```python
from build123d import *

# Parameters (mm, degrees)
SKETCH_1_W      = 100
SKETCH_1_H      = 100
SKETCH_1_R      = 1.65
EXTRUDE_1_DEPTH = 4
FILLET_1_R      = 3
SKETCH_2_W      = 9.3
SKETCH_2_H      = 10.3
EXTRUDE_2_DEPTH = 5


with BuildPart() as part:
    # 草图1 → 凸台-拉伸1 (new body)
    with BuildSketch(Plane(origin=(0, 0, 0), x_dir=(1, 0, 0), z_dir=(0, 1, 0))):
        Rectangle(SKETCH_1_W, SKETCH_1_H)
        with Locations(Location((-46, 46, 0), (0, 0, 270))):
            Circle(SKETCH_1_R, mode=Mode.SUBTRACT)
        with Locations(Location((46, 46, 0), (0, 0, 270))):
            Circle(SKETCH_1_R, mode=Mode.SUBTRACT)
        with Locations(Location((46, -46, 0), (0, 0, 270))):
            Circle(SKETCH_1_R, mode=Mode.SUBTRACT)
        with Locations(Location((-46, -46, 0), (0, 0, 270))):
            Circle(SKETCH_1_R, mode=Mode.SUBTRACT)
    extrude(amount=EXTRUDE_1_DEPTH)

    # 圆角1
    fillet_1_edges = [part.edges().sort_by_distance(p)[0] for p in [
        (50, 2, 50),
        (-50, 2, 50),
        (-50, 2, -50),
        (50, 2, -50),
    ]]
    fillet(fillet_1_edges, radius=FILLET_1_R)

    # 草图2 → 凸台-拉伸2 (add)
    with BuildSketch(Plane(origin=(0, 4, 0), x_dir=(1, 0, 0), z_dir=(0, 1, 0))):
        with Locations((52.85, -13.8)):
            Rectangle(SKETCH_2_W, SKETCH_2_H)
    extrude(amount=EXTRUDE_2_DEPTH)


solid = part.part
```
Design review of the part built by this model. Coordinates are the model's own, in mm. A direction names the side the tool comes from. Coordinates: 2 decimals unless noted, no trailing zeros. Write each loop counter-clockwise with the first axis right and the second up, starting at its lowest first coordinate (ties: lowest second). Pieces come first, ordered by that corner, then holes.
1) Machinability: for faces 5 (the flat face through (53, 6, 8.65)), 6 (the flat face through (48.2, 6, 14)), 7 (the flat face through (54, 4, 14)), which of the approach directions +Z, -Z, +X, -X, +Y, -Y give a long, thin tool a straight path to every point of the face, cutting with its end or side? Answer none if there is none.
2) Mouldability with a two-part tool opening along Z and no side actions: class faces 1 (the flat face through (53, 6, 18.95)), 2 (the cylindrical face through (-44.885, 1.972, -47.216)), 3 (the cylindrical face through (47.115, 1.972, -47.216)), 4 (the flat face through (-50, 2, 1)) as +Z half, -Z half, draft (parallel to the pull), parting line (faces both ways), or undercut.
3) To check wall thickness, follow L1, parallel to X at y = 2.95, z = 46; L2, parallel to Y at x = 8.5, z = -36.5; L3, parallel to X at y = 3, z = 25.5. State the ranges of each line that lie inside material, in increasing order.
4) Add section A-A (z = 10). Write out the cut boundary in (x, y).
5) Add section B-B (x = -7). Write out the cut boundary in (y, z), plus the area to 3 significant figures.
6) Add section C-C (z = -2.5). Write out the cut boundary in (x, y).
7) Insertion check: pin 1 (5 mm diameter, centred on x = 45, z = -19, fed in from +Y); pin 2 (1.5 mm diameter, centred on x = 53.5, y = 7.5, fed in from +Z); pin 3 (2.5 mm diameter, centred on x = 53.5, y = 7, fed in from -Z). Each pin has a flat end and moves straight along its axis. Give the tip position at first contact, or say it passes through.
Check result:
1. face 5: -Z, +X, -X, +Y
1. face 6: +Z, -Z, -X, +Y
1. face 7: +Z, -Z, +X, -Y
2. face 1: +Z half
2. face 2: undercut
2. face 3: undercut
2. face 4: draft
3. L1: x = -50 to -47.65, -44.35 to 44.35, 47.65 to 50
3. L2: y = 0 to 4
3. L3: x = -50 to 50
4. outline: (-50, 0) - (50, 0) - (50, 4) - (57.5, 4) - (57.5, 9) - (48.2, 9) - (48.2, 4) - (-50, 4) - close
5. outline: (0, -50) - (4, -50) - (4, 50) - (0, 50) - close
5. area: 400 mm2
6. outline: (-50, 0) - (50, 0) - (50, 4) - (-50, 4) - close
7. pin 1: stops at y = 4
7. pin 2: stops at z = 18.95
7. pin 3: stops at z = 8.65
